Autodesk Inventor part; units mm, degrees
ref_plane "YZ Plane" through (0, 0, 0) normal (1, 0, 0) x (0, 1, 0)
ref_plane "XZ Plane" through (0, 0, 0) normal (0, 1, 0) x (-1, 0, 0)
ref_plane "XY Plane" through (0, 0, 0) normal (0, 0, 1) x (1, 0, 0)
sketch "Sketch1" plane through (0, 0, 0) normal (0, 0, 1) x (1, 0, 0)
  line L0 (-12.1708, 16.0073) -> (13.2292, 16.0073)
  line L1 (13.2292, 16.0073) -> (13.2292, -34.7927)
  line L2 (13.2292, -34.7927) -> (-12.1708, -34.7927)
  line L3 (-12.1708, -34.7927) -> (-12.1708, 16.0073)
  line L4 (11.9592, 14.7373) -> (-10.9008, 14.7373)
  line L5 (-10.9008, 14.7373) -> (-10.9008, -33.5227)
  line L6 (-10.9008, -33.5227) -> (11.9592, -33.5227)
  line L7 (11.9592, -33.5227) -> (11.9592, 14.7373)
  point P0 (0, 0)
  dimension "d0" = 25.4
  dimension "d1" = 50.8
  dimension "d2" = 1.27
extrude "Extrusion1" add sketch "Sketch1" along normal blind 304.8
sketch "Sketch2" plane through (-12.1708, 16.0073, 0) normal (0, 1, 0) x (1, 0, 0)
  circle A0 centre (12.7, -12.7) radius 1.7272
  line L0 (25.4, 0) -> (0, 0)
  line L1 (0, 0) -> (0, -304.8)
  point P0 (12.1708, 0)
  dimension "d5" = 3.4544
  dimension "d6" = 12.7
  dimension "d7" = 12.7
extrude "Extrusion2" cut sketch "Sketch2" against normal through all
pattern_linear "Rectangular Pattern1" count 12 spacing 25.4 along (0, 0, 1) of "Extrusion2"
sketch "Sketch4" plane through (13.2292, -34.7927, 0) normal (1, 0, 0) x (0, 0, -1)
  circle A0 centre (-152.4, 25.4) radius 1.7272
  line L0 (-304.8, 0) -> (-304.8, 50.8)
  line L1 (0, 50.8) -> (-304.8, 50.8)
  point P0 (0, 34.7927)
  dimension "d21" = 3.4544
  dimension "d22" = 152.4
  dimension "d23" = 25.4
extrude "Extrusion4" cut sketch "Sketch4" against normal blind 25.4
equation "\"d3\" = d13"
equation "\"d13\" = 304.8"
properties part number "VerseFrame 12in w hole"
Geometry check sheet. Reference: the model listing, model coordinates, mm. A direction names the side the tool comes from. Give positions to 0.01 mm unless a question says otherwise; leave off trailing zeros. Loops run counter-clockwise (first coordinate to the right, second up) from the corner with the lowest first, then second, coordinate; pieces in that order, holes last.
(1) Section check C-C on x = -7.25. Record the cut outline in (y, z), then the cut area to 3 significant figures.
From the geometry:
outline: (-34.79, 0) - (-33.52, 0) - (-33.52, 304.8) - (-34.79, 304.8) - close; (14.74, 0) - (16.01, 0) - (16.01, 304.8) - (14.74, 304.8) - close
area: 774 mm2
(2) Section check B-B on y = -14. Record the cut outline in (x, z), then the cut area to 3 significant figures.
From the geometry:
outline: (-12.17, 0) - (-10.9, 0) - (-10.9, 304.8) - (-12.17, 304.8) - close; (11.96, 0) - (13.23, 0) - (13.23, 304.8) - (11.96, 304.8) - close
area: 774 mm2
(3) Section check A-A on z = 48. Record the cut outline in (x, y).
From the geometry:
outline: (-12.17, -34.79) - (13.23, -34.79) - (13.23, 16.01) - (-12.17, 16.01) - close; hole (-10.9, -33.52) - (11.96, -33.52) - (11.96, 14.74) - (-10.9, 14.74) - close
(4) Thickness scan on L1, parallel to X at y = -5.5, z = 206; L2, parallel to Y at x = 11.5, z = 131; L3, parallel to X at y = -34.25, z = 292.1. Record the ranges inside material, lowest first.
From the geometry:
L1: x = -12.17 to -10.9, 11.96 to 13.23
L2: y = -34.79 to -33.52, 14.74 to 16.01
L3: x = -12.17 to -1.2, 2.26 to 13.23
(5) Depth check by flat-ended pin: pin 1 Ø5.5 at (x, z) = (0.53, 292.1) entering from +Y. Enter the tip coordinate at first touch or a pass-through.
From the geometry:
pin 1: stops at y = 16.01
(6) Set-up check for faces 1 (the flat face through (-12, -9, 304.8)), 2 (the flat face through (11.959, -10, 150)): record each of +Z, -Z, +X, -X, +Y, -Y from which the full face is reachable in a straight line by a thin tool's end or side.
From the geometry:
face 1: +Z, +X, -X, +Y, -Y
face 2: +Z, -Z
(7) Release check for a two-part mould opening along X. For faces 3 (the flat face through (0, -33.523, 150)), 4 (the flat face through (1, -34.793, 150)), 5 (the flat face through (13.229, -9, 150)) record: released by +X, released by -X, zero draft, split by the parting line, or undercut.
From the geometry:
face 3: undercut
face 4: zero draft
face 5: released by +X
